Build history of the part. All positions in model axes, mm. A direction names the side the tool comes from. Give positions to 0.01 mm unless a question says otherwise; leave off trailing zeros. Write each loop counter-clockwise with the first axis right and the second up, starting at its lowest first coordinate (ties: lowest second). Pieces come first, ordered by that corner, then holes. Notation, with made-up numbers: (55, 36.25) -> (85, 36.25) arc R21 ccw to (85, 49.25) -> close; hole circle Ø8 at (11, -40). An arc over 180 degrees is marked (long way). Put each result on its own line as item: value.
from build123d import *

# Parameters (mm, degrees)
F0_W     = 76.2
F0_H     = 76.2
F1_DEPTH = 127
F3_DEPTH = 76.201
F4_W     = 16.764
F4_H     = 76.2
F5_DEPTH = 3.175
F7_DEPTH = 76.201


with BuildPart() as f1:
    # F0 (on Top) → F1 (new body)
    with BuildSketch(Plane.XY):
        with Locations((-0.143903846, 10.1010264666)):
            Rectangle(F0_W, F0_H)
    extrude(amount=F1_DEPTH)

    # F2 (on face) → F3 (cut, through all)
    with BuildSketch(Plane.XZ.offset(27.9989735334)):
        Polygon((37.956096154, 127), (-38.243903846, 127), (37.956096154, 105.2891537547), align=None)
    extrude(amount=-F3_DEPTH, mode=Mode.SUBTRACT)

    # F4 (on face) → F5 (join)
    with BuildSketch(Plane(origin=(30.5963615899, 0, 107.3860837485), x_dir=(0.9617256613, 0, -0.2740141465), z_dir=(0.2740141465, 0, 0.9617256613))):
        with Locations((-63.1979403185, 10.1010264666)):
            Rectangle(F4_W, F4_H)
        with Locations((-0.7293659272, 10.1010264666)):
            Rectangle(F4_W, F4_H)
    extrude(amount=F5_DEPTH)

    # F6 (on face) → F7 (cut, through all)
    with BuildSketch(Plane.XZ.offset(27.9989735334)):
        Polygon((37.956096154, 108.590511021), (37.956096154, 105.2891537547), (38.826091069, 108.3426327292), align=None)
    extrude(amount=-F7_DEPTH, mode=Mode.SUBTRACT)


solid = f1.part
1) Slice it at B-B (x = 12). Write the cut outline in (y, z), plus the area to 3 significant figures.
Filled sheet:
outline: (-28, 0) -> (48.2, 0) -> (48.2, 112.68) -> (-28, 112.68) -> close
area: 8,590 mm2
2) Pull direction Z, two halves, no side cores. Call faces 3 (the flat face through (-1, 11, 0)), 4 (the flat face through (-4, -27.999, 54)), 5 (the flat face through (-21.693, 9.568, 123.912)): released by +Z, released by -Z, zero draft, split by the parting line, or undercut.
Filled sheet:
face 3: released by -Z
face 4: zero draft
face 5: undercut
3) Wall check: L1, parallel to Z at x = 31, y = 32; L2, parallel to Z at x = 24, y = 19. Give the ranges that are in metal, low to high.
Filled sheet:
L1: 0 to 110.57
L2: 0 to 112.57
4) Pin check, flat tips, straight feed: pin 1 (2 mm diameter, centred on x = 4, y = 2.5, fed in from +Z); pin 2 (8 mm diameter, centred on x = 17.5, z = 116.5, fed in from -Y); pin 3 (2 mm diameter, centred on x = -2, y = -1, fed in from +Z). Stop position of each tip, or through.
Filled sheet:
pin 1: z = 115.25
pin 2: through
pin 3: z = 116.96
5) Tool access for faces 1 (the flat face through (22.263, 9.568, 111.388)), 2 (the flat face through (-38.244, 10, 63)): list every direction of +Z, -Z, +X, -X, +Y, -Y with a clear straight run to the whole face (end or side of a thin tool).
Filled sheet:
face 1: +Z, +Y, -Y
face 2: +Z, -Z, -X, +Y, -Y
6) Slice it at A-A (y = 0.5). Write the cut outline in (x, z).
Filled sheet:
outline: (-38.24, 0) -> (37.96, 0) -> (37.96, 108.59) -> (22.7, 112.94) -> (21.83, 109.88) -> (-22.12, 122.41) -> (-21.25, 125.46) -> (-37.37, 130.05) -> (-38.24, 127) -> close
7) Slice it at C-C (x = -14.5). Write the cut outline in (y, z).
Filled sheet:
outline: (-28, 0) -> (48.2, 0) -> (48.2, 120.23) -> (-28, 120.23) -> close
